Study the drawing (mm; zero at the part's minimum x, y, z) and answer. A direction names the side the tool comes from. Coordinates: 2 decimals unless noted, no trailing zeros. Order: outer loops, then holes, each group sorted by start corner. A loop starts at its lowest first (then second) coordinate and runs counter-clockwise, first axis right, second up. Notation, with made-up numbers: (75.25, 84.5) - (122.25, 84.5) arc R35 cw to (122.25, 116.5) - close; hole circle Ø4 at (-11.5, -37). An arc over 180 degrees is marked (long way). Write item = value, one per line.
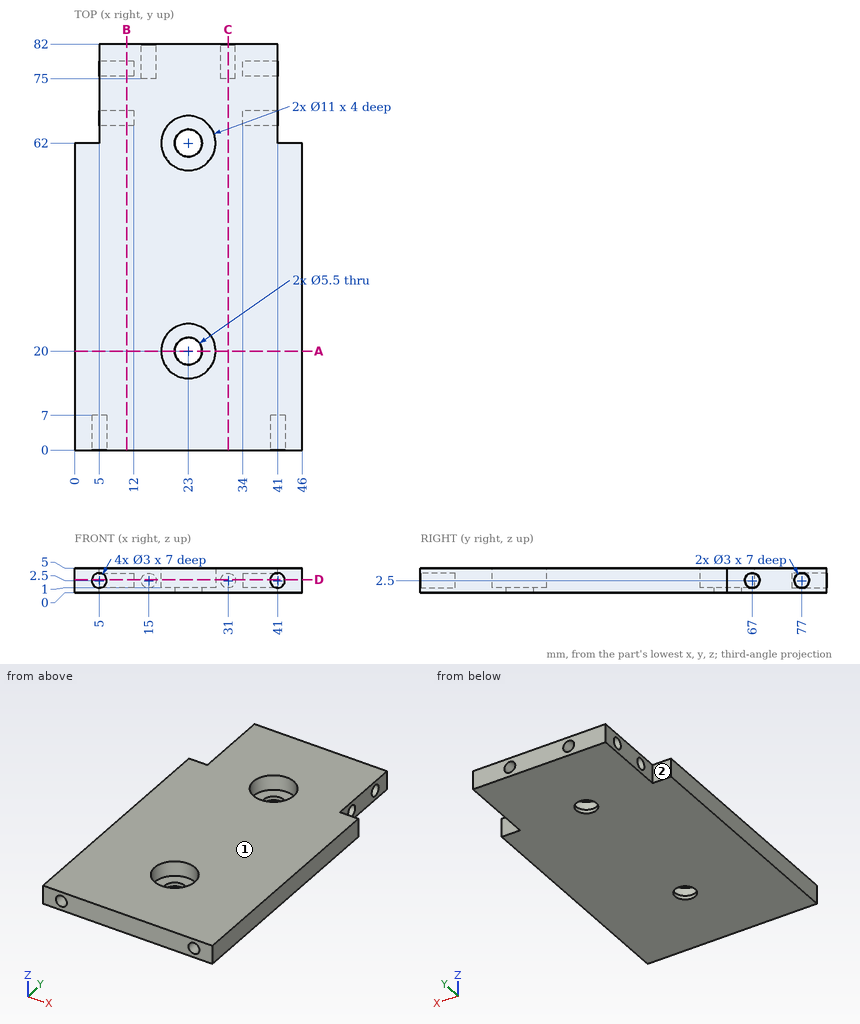
1) The part is cut by section B-B (x = 10.5). Determine the outline of the cut face in (y, z), and give its area (3 significant figures).
Returned:
outline = (0, 0) - (82, 0) - (82, 5) - (0, 5) - close; hole circle Ø3 at (67, 2.5); hole circle Ø3 at (77, 2.5)
area = 396 mm^2
2) The part is cut by section A-A (y = 20). Determine the outline of the cut face in (x, z), and give its area (4 significant figures).
Returned:
outline = (0, 0) - (20.25, 0) - (20.25, 1) - (17.5, 1) - (17.5, 5) - (0, 5) - close; (25.75, 0) - (46, 0) - (46, 5) - (28.5, 5) - (28.5, 1) - (25.75, 1) - close
area = 180.5 mm^2
3) The part is cut by section D-D (z = 2.7). Count the separate pieces of the cut face and the enclosed holes in it, and give its area (3 significant figures).
Returned:
separate_pieces = 1
enclosed_holes = 2
area = 3,220 mm^2
4) The part is cut by section C-C (x = 31). Determine the outline of the cut face in (y, z), and give its area (3 significant figures).
Returned:
outline = (0, 0) - (82, 0) - (82, 1) - (75, 1) - (75, 4) - (82, 4) - (82, 5) - (0, 5) - close
area = 389 mm^2
5) For the marked faces 1 and 2, determine the directions among +Z, -Z, +X, -X, +Y, -Y from which every point of the face is accessible in a straight line to the end or side of a thin tool.
Returned:
face_1 = +Z, +X, -X, +Y, -Y
face_2 = +Z, -Z, -X, +Y
6) Flat-ended cylindrical pins translate along their axes: pin 1 Ø1.5 at (x, z) = (44.5, 2) entering from +Y; pin 2 Ø3.5 at (x, y) = (24.5, 20) entering from +Z; pin 3 Ø2.5 at (x, z) = (41, 2.5) entering from -Y. Find the tip coordinate at first contact, or state that the pin passes through.
Returned:
pin_1 = 62
pin_2 = 1
pin_3 = 7
7) Straight lines are drawn through the part: line 1 along Y through (x, z) = (37.5, 2.5); line 2 along Y through (x, z) = (23, 1.85); line 3 along X through (y, z) = (76.5, 2.5). For each, find the intervals that lie inside material, in ascending order. Write a range as from..to.
Returned:
line_1 = 0..65.5, 68.5..75.5, 78.5..82
line_2 = 0..14.5, 25.5..56.5, 67.5..82
line_3 = 12..13.5, 16.5..29.5, 32.5..34
